Input: part model. Units: mm. Frame: model coordinates. Face numbers are marked on the shaded views. A direction names the side the tool comes from. Coordinates: 2 decimals unless noted, no trailing zeros. Write each loop counter-clockwise with the first axis right and the second up, starting at its lowest first coordinate (ties: lowest second). Pieces come first, ordered by that corner, then holes.
1) Section query C-C (y = 18.5). Output: boundary loops of the cut face in (x, z).
2) Section query B-B (y = -12.5). Output: boundary loops of the cut face in (x, z).
3) Line query: L1, parallel to Z at x = -15.5, y = 18; L2, parallel to Y at x = -7, z = -0.45; L3, parallel to X at y = 3, z = -1.1. Output: solid intervals per line, ascending.
4) Section query A-A (z = -0.8). Output: boundary loops of the cut face in (x, y), then the cut area to 3 significant figures.
5) Pin query (flat end, axial travel): pin 1 Ø0.6 at (x, z) = (1, -1) entering from +Y; pin 2 Ø1.5 at (y, z) = (-0.5, -1) entering from -X; pin 3 Ø2 at (y, z) = (8.5, -0.5) entering from +X. Return the tip coordinate at first contact, or that it passes through.
6) Set-up query: the marked faces 1 and 2. Return all of +Z, -Z, +X, -X, +Y, -Y with unobstructed straight access to the full face (end or side cutting, diameter ignored); none if empty.
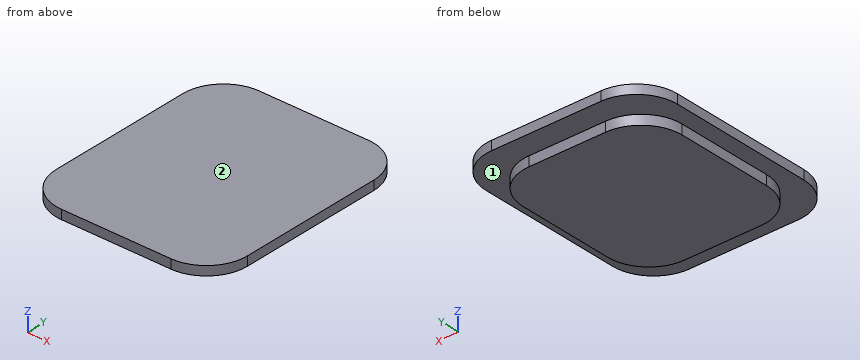
from build123d import *

# Parameters (mm, degrees)
SKETCH_2_W      = 37.34
SKETCH_2_H      = 44.43
EXTRUDE_1_DEPTH = 1.8
SKETCH_4_W      = 31
SKETCH_4_H      = 35
EXTRUDE_3_DEPTH = 1.89
FILLET_1_R      = 8
FILLET_2_R      = 8


with BuildPart() as part:
    # 草图2 → 凸台-拉伸1 (new body)
    with BuildSketch(Plane.XY):
        Rectangle(SKETCH_2_W, SKETCH_2_H)
    extrude(amount=EXTRUDE_1_DEPTH)

    # 草图4 → 凸台-拉伸3 (add)
    with BuildSketch(Plane(origin=(0, 0, 0), x_dir=(-1, 0, 0), z_dir=(0, 0, -1))):
        Rectangle(SKETCH_4_W, SKETCH_4_H)
    extrude(amount=EXTRUDE_3_DEPTH)

    # 圆角1
    fillet_1_edges = [part.edges().sort_by_distance(p)[0] for p in [
        (18.67, -22.215, 0.9),
        (-18.67, -22.215, 0.9),
        (-18.67, 22.215, 0.9),
        (18.67, 22.215, 0.9),
    ]]
    fillet(fillet_1_edges, radius=FILLET_1_R)

    # 圆角2
    fillet_2_edges = [part.edges().sort_by_distance(p)[0] for p in [
        (15.5, -17.5, -0.945),
        (-15.5, -17.5, -0.945),
        (-15.5, 17.5, -0.945),
        (15.5, 17.5, -0.945),
    ]]
    fillet(fillet_2_edges, radius=FILLET_2_R)


solid = part.part
Answer:
1. outline: (-17.43, 0) - (17.43, 0) - (17.43, 1.8) - (-17.43, 1.8) - close
2. outline: (-18.67, 0) - (-14.92, 0) - (-14.92, -1.89) - (14.92, -1.89) - (14.92, 0) - (18.67, 0) - (18.67, 1.8) - (-18.67, 1.8) - close
3. L1: z = 0 to 1.8
3. L2: y = -17.5 to 17.5
3. L3: x = -15.5 to 15.5
4. outline: (-15.5, -9.5) arc R8 ccw to (-7.5, -17.5) - (7.5, -17.5) arc R8 ccw to (15.5, -9.5) - (15.5, 9.5) arc R8 ccw to (7.5, 17.5) - (-7.5, 17.5) arc R8 ccw to (-15.5, 9.5) - close
4. area: 1,030 mm2
5. pin 1: stops at y = 17.5
5. pin 2: stops at x = -15.5
5. pin 3: stops at x = 18.67
6. face 1: -Z
6. face 2: +Z, +X, -X, +Y, -Y
